Here's how the part is built. I have some questions about the finished solid (model axes, mm). A direction names the side the tool comes from. Coordinates: 2 decimals unless noted, no trailing zeros. Order: outer loops, then holes, each group sorted by start corner. A loop starts at its lowest first (then second) coordinate and runs counter-clockwise, first axis right, second up. Notation, with made-up numbers: M -34.75,6.25 L 11.25,6.25 A20 cw 11.25,43.25 Z; hole C 83.25,58 d3. An arc over 180 degrees is marked long. One line per question, with ' | ' between items. Start each with the question number.
```python
from build123d import *

# Parameters (mm, degrees)
SKETCH1_W                       = 25.4
SKETCH1_H                       = 50.8
SKETCH1_W_2                     = 19.05
SKETCH1_H_2                     = 44.45
BOSS_EXTRUDE1_DEPTH             = 38.1
F_5_32_0_15625_DIAMETER_HOLE1_D = 3.96875
SKETCH5_R                       = 14.2875
CUT_EXTRUDE1_DEPTH              = 53.363441445


with BuildPart() as part:
    # Sketch1 → Boss-Extrude1 (new, symmetric)
    with BuildSketch(Plane(origin=(0, 0, 0), x_dir=(1, 0, 0), z_dir=(0, 1, 0))):
        Rectangle(SKETCH1_W, SKETCH1_H)
        Rectangle(SKETCH1_W_2, SKETCH1_H_2, mode=Mode.SUBTRACT)
    extrude(amount=BOSS_EXTRUDE1_DEPTH, both=True)

    # 5/32 (0.15625) Diameter Hole1 (through all)
    with Locations(Plane(origin=(0, 0, -25.4), x_dir=(-1, 0, 0), z_dir=(0, 0, -1))):
        with Locations((0, 25.4), (0, 12.7), (0, 0), (0, -12.7), (0, -25.4), (0, -38.1), (0, -50.8), (0, -63.5), (0, -76.2), (0, -88.9), (0, -101.6), (0, -114.3), (0, -127), (0, -139.7), (0, -152.4), (0, -165.1), (0, -177.8), (0, -190.5), (0, -203.2), (0, -215.9), (0, -228.6), (0, -241.3), (0, -254), (0, -266.7), (0, -279.4), (0, -292.1), (0, -304.8), (0, -317.5), (0, -330.2), (0, -342.9), (0, -355.6), (0, -368.3), (0, -381), (0, -393.7), (0, -406.4), (0, -419.1), (0, -431.8), (0, -444.5), (0, -457.2), (0, -469.9), (0, -482.6), (0, -495.3), (0, -508), (0, -520.7), (0, -533.4), (0, -546.1), (0, -558.8), (0, -571.5), (0, -584.2), (0, -596.9), (0, -609.6), (0, -622.3), (0, -635), (0, -647.7), (0, -660.4), (0, -673.1), (0, -685.8), (0, -698.5), (0, -711.2), (0, -723.9), (0, -736.6), (0, -749.3), (0, -762), (0, -774.7), (0, -787.4), (0, -800.1), (0, -812.8), (0, -825.5), (0, -838.2)):
            Hole(F_5_32_0_15625_DIAMETER_HOLE1_D / 2)

    # Sketch5 → Cut-Extrude1 (cut, through all)
    with BuildSketch(Plane(origin=(12.7, 0, 0), x_dir=(0, 0, -1), z_dir=(1, 0, 0))):
        Circle(SKETCH5_R)
    extrude(amount=-CUT_EXTRUDE1_DEPTH, mode=Mode.SUBTRACT)


solid = part.part
```
1. Will this pin go through, and if not, where does the flat tip stop? pin 1 (2.5 mm diameter, centred on x = 0, y = -25.4, fed in from -Z).
2. Imagine slicing it at B-B (y = 21). List the corners of the cut face in (x, z) for me (3 decimals), then the cut area to 3 significant figures.
3. Which directions (+Z, -Z, +X, -X, +Y, -Y) give clear straight access to the entire face, cutting with the end or side of a thin tool? Please do faces 4 (the face through (0.044, -36.116, -23.79)), 5 (the face through (-9.525, 1, 15)).
4. Imagine slicing it at D-D (y = 0). List the corners of the cut face in (x, z) for me (1 decimal).
5. We'd pull the mould along X, two halves only. Please class faces 1 (the face through (12.7, 9, 12)), 2 (the face through (-0.43, -1.937, -23.79)), 3 (the face through (3, 1, 25.4)): released by +X, released by -X, zero draft, split by the parting line, or undercut.
6. Imagine slicing it at A-A (x = -3). List the corners of the cut face in (y, z) for me (3 decimals).
7. I need wall thicknesses on line 1 (Y direction, x = 0, z = 24.1); line 2 (Z direction, x = -4, y = -35) (3 decimals); line 3 (X direction, y = -23, z = 11) (3 decimals). Which ranges of each line are inside material? Lowest first, please.
8. Imagine slicing it at C-C (z = -16). List the corners of the cut face in (x, y) for me (3 decimals), then the cut area to 3 significant figures.
Entries:
1) pin 1: through
2) outline: M -12.7,-25.4 L 12.7,-25.4 L 12.7,25.4 L -12.7,25.4 Z; hole M -9.525,-22.225 L 9.525,-22.225 L 9.525,22.225 L -9.525,22.225 Z | area: 444 mm²
3) face 4: +Z, -Z, -Y | face 5: +Y, -Y
4) outline: M -12.7,-25.4 L -2,-25.4 L -2,-22.2 L -9.5,-22.2 L -9.5,-14.3 L -12.7,-14.3 Z; M -12.7,14.3 L -9.5,14.3 L -9.5,22.2 L -2,22.2 L -2,25.4 L -12.7,25.4 Z; M 2,-25.4 L 12.7,-25.4 L 12.7,-14.3 L 9.5,-14.3 L 9.5,-22.2 L 2,-22.2 Z; M 2,22.2 L 9.5,22.2 L 9.5,14.3 L 12.7,14.3 L 12.7,25.4 L 2,25.4 Z
5) face 1: released by +X | face 2: undercut | face 3: zero draft
6) outline: M -38.1,-25.4 L 38.1,-25.4 L 38.1,-22.225 L -38.1,-22.225 Z; M -38.1,22.225 L 38.1,22.225 L 38.1,25.4 L -38.1,25.4 Z
7) line 1: -36.12 to -27.38, -23.42 to -14.68, -10.72 to -1.98, 1.98 to 10.72, 14.68 to 23.42, 27.38 to 38.1 | line 2: -25.4 to -22.225, 22.225 to 25.4 | line 3: -12.7 to -9.525, 9.525 to 12.7
8) outline: M -12.7,-38.1 L -9.525,-38.1 L -9.525,38.1 L -12.7,38.1 Z; M 9.525,-38.1 L 12.7,-38.1 L 12.7,38.1 L 9.525,38.1 Z | area: 484 mm²
